Autodesk Inventor part; units mm, degrees
ref_plane "YZ Plane" through (0, 0, 0) normal (1, 0, 0) x (0, 1, 0)
ref_plane "XZ Plane" through (0, 0, 0) normal (0, 1, 0) x (-1, 0, 0)
ref_plane "XY Plane" through (0, 0, 0) normal (0, 0, 1) x (1, 0, 0)
sketch "Sketch1" plane through (0, 0, 0) normal (0, 0, 1) x (1, 0, 0)
  circle A0 centre (0, 0) radius 80
  line L0 (37.5, 37.5) -> (-37.5, 37.5)
  line L1 (-37.5, 37.5) -> (-37.5, -37.5)
  line L2 (-37.5, -37.5) -> (37.5, -37.5)
  line L3 (37.5, -37.5) -> (37.5, 37.5)
  line L4 (37.5, 37.5) -> (-37.5, -37.5) construction
  line L5 (-37.5, 37.5) -> (37.5, -37.5) construction
  circle A1 centre (0, 0) radius 62.5 construction
  circle A2 centre (-62.5, 0) radius 8.5
  circle A3 centre (0, -62.5) radius 8.5
  circle A4 centre (62.5, 0) radius 8.5
  circle A5 centre (0, 62.5) radius 8.5
  dimension "d171" = 125
  dimension "d157" = 160
  dimension "d158" = 75
  dimension "d176" = 17
  dimension "d179" = 360
extrude "Plate5" add sketch "Sketch1" along normal blind 3
properties part number "PRS-1651 FDS MAIN  FLANGE_CPY" material "Stainless Steel"
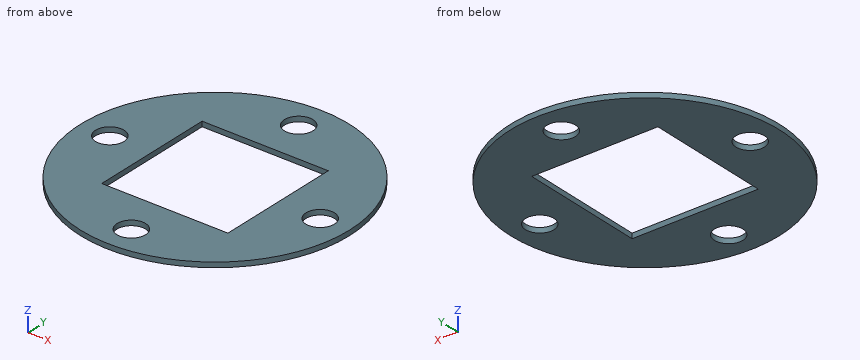
For this review, take the finished solid that the model builds, in its own axes (mm). Give positions to 0.01 mm unless a question says otherwise; leave off trailing zeros. Write each loop counter-clockwise with the first axis right and the second up, starting at its lowest first coordinate (ties: lowest second). Pieces come first, ordered by that corner, then holes.
Item 1: Insertion check: P1, Ø22, axis at x = 0, y = -62.5, coming from the +Z side; P2, Ø0.9, axis at y = -12, z = 1.5, coming from the +X side. Each pin has a flat end and moves straight along its axis. Give the tip position at first contact, or say it passes through.
Item 2: Take a section at C-C (z = 1.7). Give the boundary of the cut face in (x, y).
Item 3: Take a section at A-A (x = 0). Give the boundary of the cut face in (y, z), and give its area (3 significant figures).
Item 4: Wall thickness on probe 1 along Y at (x, z) = (0, 1.55); probe 2 along X at (y, z) = (2, 2.1) (3 decimals); probe 3 along Y at (x, z) = (3, 2.1): over which ranges is each line inside the solid? List them lowest first.
Item 5: Take a section at D-D (x = 57.5). Give the boundary of the cut face in (y, z).
Established:
1. P1: stops at z = 3
1. P2: stops at x = 79.16
2. outline: circle Ø160 at (0, 0); hole circle Ø17 at (-62.5, 0); hole (-37.5, -37.5) - (37.5, -37.5) - (37.5, 37.5) - (-37.5, 37.5) - close; hole circle Ø17 at (0, -62.5); hole circle Ø17 at (0, 62.5); hole circle Ø17 at (62.5, 0)
3. outline: (-80, 0) - (-71, 0) - (-71, 3) - (-80, 3) - close; (-54, 0) - (-37.5, 0) - (-37.5, 3) - (-54, 3) - close; (37.5, 0) - (54, 0) - (54, 3) - (37.5, 3) - close; (71, 0) - (80, 0) - (80, 3) - (71, 3) - close
3. area: 153 mm2
4. probe 1: y = -80 to -71, -54 to -37.5, 37.5 to 54, 71 to 80
4. probe 2: x = -79.975 to -70.761, -54.239 to -37.5, 37.5 to 54.239, 70.761 to 79.975
4. probe 3: y = -79.94 to -70.45, -54.55 to -37.5, 37.5 to 54.55, 70.45 to 79.94
5. outline: (-55.62, 0) - (-6.87, 0) - (-6.87, 3) - (-55.62, 3) - close; (6.87, 0) - (55.62, 0) - (55.62, 3) - (6.87, 3) - close
